CAD build for the part. Positions are in the model's coordinates, mm. A direction names the side the tool comes from. Coordinates: 2 decimals unless noted, no trailing zeros. Write each loop counter-clockwise with the first axis right and the second up, starting at its lowest first coordinate (ties: lowest second). Pieces come first, ordered by that corner, then holes. Notation, with made-up numbers: (-3, -37.75) - (30, -37.75) arc R18 ccw to (30, -25.75) - close; hole circle Ø4 at (26.5, 54.5). An arc over 180 degrees is marked (long way). One line per question, with ' | ' between items. Start each with the question number.
1. Which spindle directions (+Z, -Z, +X, -X, +Y, -Y) get a long thin tool onto all of the face, cutting with end or side? Do faces 4 (the flat face through (0.514, -51.255, -0.751)), 5 (the flat face through (-9.226, -51.745, 23.006)), 6 (the flat face through (-7, 0, 27)), 7 (the flat face through (-7.76, -4.44, 25.86)), 8 (the flat face through (-7.3, -51.74, -2.58)). Say none if no direction does.
2. Probe line 1 (Y direction, x = -9.5, z = -27.5); line 2 (Y direction, x = -2, z = -21); line 3 (Z direction, x = -19, y = -8.5). List the from-to ranges inside material, lowest first.
3. Band-saw the part on C-C, the plane y = -35. Write the cut outline in (x, z).
4. Band-saw the part on D-D, the plane z = 26. Write the cut outline in (x, y), then the cut area to 3 significant figures.
5. Band-saw the part on B-B, the plane x = 20.5. Write the cut outline in (y, z), then the cut area to 3 significant figures.
6. Band-saw the part on A-A, the plane y = -5.5. Write the cut outline in (x, z), then the cut area to 3 significant figures.
7. Two-plate mould, pull along Z, no slides. Class faces 1 (the cylindrical face through (31, -16.76, 9.76)), 2 (the flat face through (21, -24, -10)), 3 (the flat face through (2.38, -51.26, -25.63)): +Z half, -Z half, draft (parallel to the pull), parting line (faces both ways), or undercut.
8. Flat gauge pins, fed straight in: P1, Ø3, axis at x = -16, y = -45, coming from the +Z side; P2, Ø4, axis at x = -2, z = -21.5, coming from the +Y side; P3, Ø8, axis at y = -49, z = 1, coming from the -X side; P4, Ø1.5, axis at x = 12.5, z = 21, coming from the +Y side. Where does each tip first touch, or does it go through?
from build123d import *

# Parameters (mm, degrees)
F0_R      = 32.5
F1_DEPTH  = 9
F2_R      = 32.5
F3_DEPTH  = 25
F6_DEPTH  = 35
F8_DEPTH  = 35
F10_DEPTH = 25
F11_R     = 2.5
F12_DEPTH = 25
F13_R     = 2.5
F14_DEPTH = 15


with BuildPart() as f1:
    # F0 (on Front) → F1 (new body)
    with BuildSketch(Plane.XZ):
        Circle(F0_R)
        with BuildLine():
            ThreePointArc((6.0477952292, 29.8943836341), (8.5507887297, -29.2768511302), (-21.1868965868, 21.9400413177))
            Line((-21.1868965868, 21.9400413177), (6.0477952292, 29.8943836341))
        make_face(mode=Mode.SUBTRACT)
    extrude(amount=F1_DEPTH)

    # F2 (on face) → F3 (join)
    with BuildSketch(Plane.XZ.offset(9)):
        Circle(F2_R)
    extrude(amount=F3_DEPTH)

    # F5 (on face) → F6 (join)
    with BuildSketch(Plane.XZ.offset(34)):
        with BuildLine():
            Line((7.7129205553, -31.5715197054), (-7.0699844214, 31.7216853317))
            ThreePointArc((-7.0699844214, 31.7216853317), (-31.6482352223, -7.3918338264), (7.7129205553, -31.5715197054))
        make_face()
    extrude(amount=F6_DEPTH)

    # F7 (on face) → F8 (cut)
    with BuildSketch(Plane.XZ.offset(69)):
        with BuildLine():
            Line((0, -32.5), (-14.9713811536, 28.8462778596))
            ThreePointArc((-14.9713811536, 28.8462778596), (-31.5733592641, -7.705386738), (0, -32.5))
        make_face()
    extrude(amount=-F8_DEPTH, mode=Mode.SUBTRACT)

    # F9 (on face) → F10 (cut)
    with BuildSketch(Plane(origin=(0.321468067, 0, 0.0750828131), x_dir=(0, 1, 0), z_dir=(0.973791853, 0, 0.2274410408))):
        Polygon((-34, -40.3801463544), (-34, -32.4983233545), (-34, -25.4983233545), (-69, -25.4983233545), (-69, -32.4983233545), (-69, -40.3801463544), align=None)
        Polygon((-69, 32.4983233545), (-69, 24.5016766455), (-34, 24.5016766455), (-34, 32.4983233545), (-34, 45.2751591802), (-69, 45.2751591802), align=None)
    extrude(amount=-F10_DEPTH, mode=Mode.SUBTRACT)

    # F11 (on face) → F12 (cut)
    with BuildSketch(Plane(origin=(0.321468067, 0, 0.0750828131), x_dir=(0, 1, 0), z_dir=(0.973791853, 0, 0.2274410408))):
        with Locations((-50, -13.7305416178)):
            Circle(F11_R)
        with Locations((-50.3844208735, 13.2694583822)):
            Circle(F11_R)
    extrude(amount=-F12_DEPTH, mode=Mode.SUBTRACT)

    # F13 (on face) → F14 (cut)
    with BuildSketch(Plane(origin=(0, -9, 0), x_dir=(-1, 0, 0), z_dir=(0, 1, 0))):
        with Locations((-20.5235508249, -9.6324379852)):
            Circle(F13_R)
        with Locations((-11.8325852307, 20.1243615242)):
            Circle(F13_R)
        with Locations((14.2461454022, 16.6747516077)):
            Circle(F13_R)
        with Locations((3.0319962484, -21.7211187269)):
            Circle(F13_R)
    extrude(amount=-F14_DEPTH, mode=Mode.SUBTRACT)


solid = f1.part
Filled in:
1) face 4: +Z, +X, -Y | face 5: +Z, -X, -Y | face 6: +Z, -Z, +X, -X, +Y | face 7: +Y | face 8: -Z, -X, -Y
2) line 1: y = -34 to -9 | line 2: y = -69 to -24 | line 3: z = -26.37 to -23.86, 22.58 to 26.37
3) outline: (-13.31, 22.05) - (-1.46, -26.53) - (6.12, -24.75) - (-5.25, 23.93) - close
4) outline: (-19.5, -34) - (19.5, -34) - (19.5, 0) - (15.95, 0) - (15.95, -9) - (-7.29, -9) - (-7.29, 0) - (-19.5, 0) - close | area: 1,120 mm²
5) outline: (-34, -25.22) - (0, -25.22) - (0, -22.58) - (-9, -22.58) - (-9, -12.13) - (-24, -12.13) - (-24, -7.13) - (-9, -7.13) - (-9, 22.58) - (0, 22.58) - (0, 25.22) - (-34, 25.22) - close | area: 1,230 mm²
6) outline: circle Ø65 at (0, 0); hole (-21.19, 21.94) arc R30.5 ccw (long way) to (6.05, 29.89) - close | area: 463 mm²
7) face 1: parting line | face 2: undercut | face 3: -Z half
8) P1: passes through | P2: stops at y = -9 | P3: stops at x = -9.15 | P4: stops at y = -24
